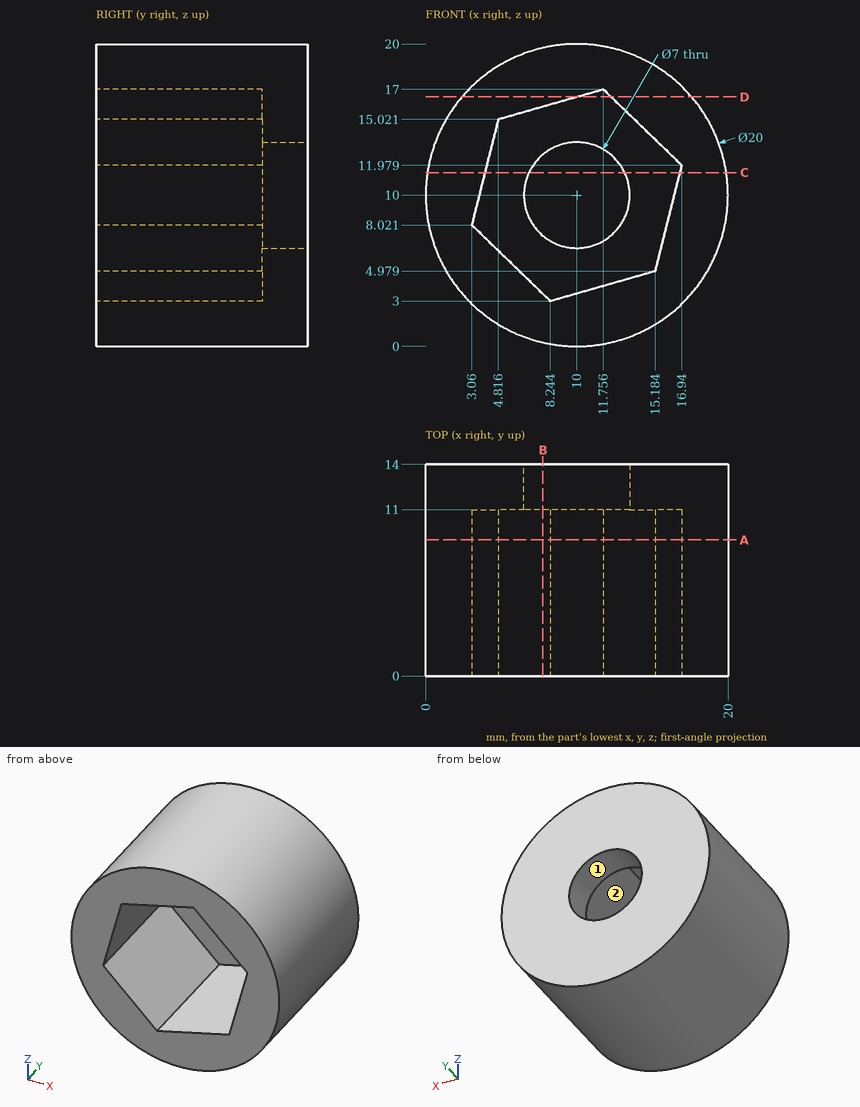
Print and shaded views of the part. All mm, measured from the part's lowest x, y and z. A direction names the side the tool comes from. Give positions to 0.01 mm unless a question says otherwise; leave off trailing zeros. Order: outer loops, then holes, each group sorted by start corner. A loop starts at its lowest first (then second) coordinate and runs counter-clockwise, first axis right, second up. Notation, with made-up numbers: (62, 4.5) - (113, 4.5) arc R10 ccw to (113, 20.5) - close; hole circle Ø1 at (44.5, 14). An arc over 180 degrees is marked (long way). Use a Markdown table: item, result.
1) Probe L1, parallel to Z at x = 10, y = 11.7; L2, parallel to Y at x = 10.25, z = 14.25; L3, parallel to X at y = 3, z = 9.5. List the from-to ranges inside material, lowest first. Write a range as from..to.
Checked values:
| item | result |
|---|---|
| L1 | 0..6.5, 13.5..20 |
| L2 | 11..14 |
| L3 | 0.01..3.43, 16.32..19.99 |
2) Saw through at C-C on z = 11.5. List the corners of the cut face in (x, y).
Checked values:
| item | result |
|---|---|
| outline | (0.11, 0) - (3.93, 0) - (3.93, 11) - (6.84, 11) - (6.84, 14) - (0.11, 14) - close; (13.16, 11) - (16.82, 11) - (16.82, 0) - (19.89, 0) - (19.89, 14) - (13.16, 14) - close |
3) Flat gauge pins, fed straight in: P1, Ø1.5, axis at y = 6, z = 11, coming from the +X side; P2, Ø5, axis at y = 2, z = 13.5, coming from the -X side; P3, Ø3, axis at x = 4, y = 4.5, coming from the -Z side. Where does each tip first touch, or does it go through?
Checked values:
| item | result |
|---|---|
| P1 | x = 20 |
| P2 | x = 0.05 |
| P3 | z = 1.07 |
4) Saw through at D-D on z = 16.5. List the corners of the cut face in (x, y).
Checked values:
| item | result |
|---|---|
| outline | (2.4, 0) - (10, 0) - (10, 11) - (12.27, 11) - (12.27, 0) - (17.6, 0) - (17.6, 14) - (2.4, 14) - close |
5) Saw through at B-B on x = 7.75. List the corners of the cut face in (y, z), plus the area to 3 significant figures.
Checked values:
| item | result |
|---|---|
| outline | (0, 0.26) - (14, 0.26) - (14, 7.32) - (11, 7.32) - (11, 3.48) - (0, 3.48) - close; (0, 15.86) - (11, 15.86) - (11, 12.68) - (14, 12.68) - (14, 19.74) - (0, 19.74) - close |
| area | 121 mm² |
6) Saw through at A-A on y = 9. List the corners of the cut face in (x, z).
Checked values:
| item | result |
|---|---|
| outline | circle Ø20 at (10, 10); hole (3.06, 8.02) - (8.24, 3) - (15.18, 4.98) - (16.94, 11.98) - (11.76, 17) - (4.82, 15.02) - close |
7) 3-axis set-ups, long thin cutter, end or side, ignore diameter. For the marked faces 1 and 2: which of +Z, -Z, +X, -X, +Y, -Y reach the whole face in a straight line?
Checked values:
| item | result |
|---|---|
| face 1 | +Y, -Y |
| face 2 | -Y |
